The listing builds one solid part. Answer for the finished solid, in the listing's coordinates (mm). A direction names the side the tool comes from. Round coordinates to 2 decimals unless told otherwise and drop trailing zeros. Loops run counter-clockwise (first coordinate to the right, second up) from the corner with the lowest first, then second, coordinate; pieces in that order, holes last. Notation, with made-up numbers: (-22.5, -25) -> (22.5, -25) arc R18 cw to (22.5, 4) -> close; hole circle Ø1 at (40.25, 50). An arc over 180 degrees is marked (long way). One line per question, with ' | ' between items.
from build123d import *

# Parameters (mm, degrees)
F1_DEPTH = 5.08


with BuildPart() as f1:
    # F0 (on Top) → F1 (new body)
    with BuildSketch(Plane.XY):
        Polygon((16.09368, 17.915163), (-15.924582, 17.915163), (-31.849165, 0), (0, -32.017816), (32.18736, 0), align=None)
        Polygon((0, -26.889354), (-24.409898, -2.350199), (-17.397631, -2.360984), (0, -19.850741), (17.528368, -2.414702), (24.747919, -2.425806), align=None, mode=Mode.SUBTRACT)
        with BuildLine():
            ThreePointArc((-15.731339, 10.879274), (-4.832174, 12.101478), (-9.286881, 2.079444))
            ThreePointArc((-9.286881, 2.079444), (-9.959517, 8.346525), (-15.731339, 10.879274))
        make_face(mode=Mode.SUBTRACT)
        with BuildLine():
            ThreePointArc((2.155719, 9.712794), (13.510836, 12.771188), (10.564446, 1.386495))
            ThreePointArc((10.564446, 1.386495), (8.75362, 7.966877), (2.155719, 9.712794))
        make_face(mode=Mode.SUBTRACT)
    extrude(amount=F1_DEPTH)


solid = f1.part
Q1. A cutting plane is placed at C-C on z = 1.75. Give the vertices of the cut face in (x, y).
Numbers:
outline: (-31.85, 0) -> (0, -32.02) -> (32.19, 0) -> (16.09, 17.92) -> (-15.92, 17.92) -> close; hole (-24.41, -2.35) -> (0, -26.89) -> (24.75, -2.43) -> (17.53, -2.41) -> (0, -19.85) -> (-17.4, -2.36) -> close; hole (-15.73, 10.88) arc R6.29 cw to (-9.29, 2.08) arc R6.32 ccw (long way) to start; hole (2.16, 9.71) arc R6.85 cw to (10.56, 1.39) arc R6.8 ccw (long way) to start
Q2. Find the intervals of material crossed by line 1 (Y direction, x = -12, z = 3); line 2 (Y direction, x = -14.5, z = 2.6); line 3 (X direction, y = -18, z = 1.5), in increasing order. Write a range as from..to.
Numbers:
line 1: -19.95..-14.83, -7.79..10.14, 14.34..17.92 | line 2: -17.44..-12.31, -5.27..10.9, 12.73..17.92 | line 3: -13.94..-8.84, -1.84..1.86, 8.99..14.09
Q3. For faces 4 (the face through (8.641, -11.255, 2.504)), 5 (the face through (-16.15, -15.78, 2.5)), determine the directions among +Z, -Z, +X, -X, +Y, -Y from which every point of the face is accessible in a straight line to the end or side of a thin tool.
Numbers:
face 4: +Z, -Z | face 5: +Z, -Z, -X, -Y
Q4. A cutting plane is placed at D-D on y = -11.5. Give the vertices of the cut face in (x, z), plus the area to 3 significant figures.
Numbers:
outline: (-20.41, 0) -> (-15.31, 0) -> (-15.31, 5.08) -> (-20.41, 5.08) -> close; (-8.31, 0) -> (8.39, 0) -> (8.39, 5.08) -> (-8.31, 5.08) -> close; (15.57, 0) -> (20.63, 0) -> (20.63, 5.08) -> (15.57, 5.08) -> close | area: 136 mm^2
Q5. Given pin 1 Ø1.5 at (x, y) = (-19.5, -14.5) entering from +Z; pin 2 Ø3 at (x, z) = (23, 3) entering from -Y; pin 3 Ø1.5 at (y, z) = (-7.5, 4) entering from +X, each flat-ended and moving along its own axis, determine where each tip first touches the part or whether it passes through.
Numbers:
pin 1: through | pin 2: y = -10.63 | pin 3: x = 25.4
Q6. For a pull along Y with two mould halves and no side action, classify faces 1 (the face through (12.547, -14.486, 2.504)), 2 (the face through (15.9, -16.2, 2.5)), 3 (the face through (0, 17.915, 3)) as pulls with the +Y half, pulls with the -Y half, needs draft (parallel to the pull), parting line crosses it, or undercut.
Numbers:
face 1: undercut | face 2: pulls with the -Y half | face 3: pulls with the +Y half
Q7. A cutting plane is placed at B-B on y = -22. Give the vertices of the cut face in (x, z).
Numbers:
outline: (-9.97, 0) -> (-4.86, 0) -> (-4.86, 5.08) -> (-9.97, 5.08) -> close; (4.95, 0) -> (10.07, 0) -> (10.07, 5.08) -> (4.95, 5.08) -> close
Q8. A cutting plane is placed at A-A on x = 3.5. Give the vertices of the cut face in (y, z).
Numbers:
outline: (-28.54, 0) -> (-23.43, 0) -> (-23.43, 5.08) -> (-28.54, 5.08) -> close; (-16.37, 0) -> (9.93, 0) -> (9.93, 5.08) -> (-16.37, 5.08) -> close; (12.3, 0) -> (17.92, 0) -> (17.92, 5.08) -> (12.3, 5.08) -> close
